from build123d import *

# Parameters (mm, degrees)
BOSS_EXTRUDE1_DEPTH     = 2
BOSS_EXTRUDE2_DEPTH     = 5.4
CUT_EXTRUDE2_DEPTH      = 324.312541101
CUT_EXTRUDE2_DEPTH_BACK = 324.312541101
SKETCH11_R              = 3.15
SKETCH11_R_2            = 8.5
SKETCH13_R              = 3.289472506
BOSS_EXTRUDE3_DEPTH     = 3


with BuildPart() as part:
    # Sketch3 → Boss-Extrude1 (new body)
    with BuildSketch(Plane(origin=(0, 0, 0), x_dir=(1, 0, 0), z_dir=(0, 1, 0))):
        with BuildLine():
            ThreePointArc((271.153533245, 18.921159404), (199.331937646, 37.525228411), (127.510342047, 18.921159404))
            ThreePointArc((127.510342047, 18.921159404), (108.90627304, -52.900436194), (127.510342047, -124.722031793))
            ThreePointArc((127.510342047, -124.722031793), (199.331937646, -143.3261008), (271.153533245, -124.722031793))
            ThreePointArc((271.153533245, -124.722031793), (289.757602252, -52.900436194), (271.153533245, 18.921159404))
        make_face()
    extrude(amount=BOSS_EXTRUDE1_DEPTH)

    # Sketch5 → Boss-Extrude2 (add)
    with BuildSketch(Plane(origin=(0, 2, 0), x_dir=(1, 0, 0), z_dir=(0, 1, 0))):
        with BuildLine():
            Line((121.611565862, -109.080289564), (120.36423024, -109.98653194))
            ThreePointArc((120.36423024, -109.98653194), (108.906273045, -52.899217103), (120.365171108, 4.187908885))
            Line((120.365171108, 4.187908885), (121.612501818, 3.281670078))
            ThreePointArc((121.612501818, 3.281670078), (110.406273045, -52.899216401), (121.611565862, -109.080289564))
        make_face()
        with BuildLine():
            Line((143.152084277, -130.620807978), (142.2458419, -131.8681436))
            ThreePointArc((142.2458419, -131.8681436), (199.331937646, -143.3261008), (256.418033392, -131.8681436))
            Line((256.418033392, -131.8681436), (255.511791015, -130.620807978))
            ThreePointArc((255.511791015, -130.620807978), (199.331937646, -141.8261008), (143.152084277, -130.620807978))
        make_face()
        with BuildLine():
            Line((277.052309429, 3.279417175), (278.299645052, 4.185659552))
            ThreePointArc((278.299645052, 4.185659552), (289.757602252, -52.900436194), (278.299645052, -109.98653194))
            Line((278.299645052, -109.98653194), (277.052309429, -109.080289564))
            ThreePointArc((277.052309429, -109.080289564), (288.257602252, -52.900436194), (277.052309429, 3.279417175))
        make_face()
        with BuildLine():
            Line((255.511791015, 24.819935589), (256.418033392, 26.067271212))
            ThreePointArc((256.418033392, 26.067271212), (199.330718555, 37.525228406), (142.243592567, 26.066330343))
            Line((142.243592567, 26.066330343), (143.149831374, 24.818999633))
            ThreePointArc((143.149831374, 24.818999633), (199.330717853, 36.025228406), (255.511791015, 24.819935589))
        make_face()
    extrude(amount=BOSS_EXTRUDE2_DEPTH)

    # Sketch11 → Cut-Extrude2 (cut, two sides: drawn at the far end of the back side and taken through both)
    with BuildSketch(Plane(origin=(0, 2, 0), x_dir=(1, 0, 0), z_dir=(0, 1, 0)).offset(-CUT_EXTRUDE2_DEPTH_BACK)):
        with Locations(Location((171.047666398, -24.616164947, 0), (0, 0, 270))):
            Circle(SKETCH11_R)
        with Locations(Location((227.616208893, -24.616164947, 0), (0, 0, 270))):
            Circle(SKETCH11_R)
        with Locations(Location((227.616208893, -81.184707442, 0), (0, 0, 270))):
            Circle(SKETCH11_R)
        with Locations(Location((171.047666398, -81.184707442, 0), (0, 0, 270))):
            Circle(SKETCH11_R)
        with Locations(Location((199.331937646, -75.900436194, 0), (0, 0, 270))):
            Circle(SKETCH11_R_2)
    extrude(amount=CUT_EXTRUDE2_DEPTH + CUT_EXTRUDE2_DEPTH_BACK, mode=Mode.SUBTRACT)

    # Sketch13 → Boss-Extrude3 (add)
    with BuildSketch(Plane(origin=(0, 2, 0), x_dir=(1, 0, 0), z_dir=(0, 1, 0))):
        with Locations(Location((189.331937646, -85.900436194, 0), (0, 0, 270))):
            Circle(SKETCH13_R)
        with Locations(Location((209.331937646, -85.900436194, 0), (0, 0, 270))):
            Circle(SKETCH13_R)
    extrude(amount=BOSS_EXTRUDE3_DEPTH)


solid = part.part
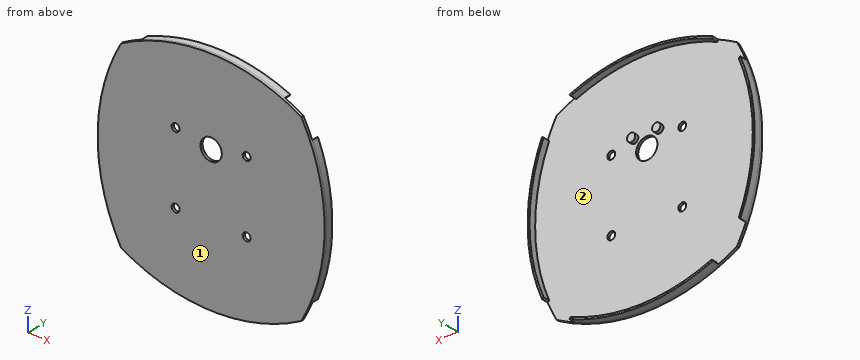
CAD build for the part. Positions are in the model's coordinates, mm. Face numbers are marked on the shaded views. Round coordinates to 2 decimals unless told otherwise and drop trailing zeros. Loops run counter-clockwise (first coordinate to the right, second up) from the corner with the lowest first, then second, coordinate; pieces in that order, holes last.
(1) Wall check: line 1 along Z through (x, y) = (169.5, 1.5); line 2 along X through (y, z) = (6, 50) (3 decimals); line 3 along Z through (x, y) = (187, 3.5). Give the ranges that are in metal, low to high.
(2) Cut at D-D (z = 2). Give the cut face in (x, y).
(3) Drop flat-ended pins along their axis: pin 1 (12 mm diameter, centred on x = 270.5, z = 42.5, fed in from +Y); pin 2 (4 mm diameter, centred on x = 227.62, z = 24.62, fed in from -Y); pin 3 (3.5 mm diameter, centred on x = 208, z = 87, fed in from +Y); pin 4 (2 mm diameter, centred on y = 6, z = 7.5, fed in from -X). Give the stop position or say it passes through.
(4) Cut at B-B (z = 73). Give the cut face in (x, y), plus the area to 3 significant figures.
(5) Cut at A-A (y = 3.5). Give the cut face in (x, z), plus the area to 3 significant figures.
(6) Cut at C-C (x = 250). Give the cut face in (y, z).
(7) Two-plate mould, pull along X, no slides. Class the marked faces 1 and 2: +X half, -X half, draft (parallel to the pull), parting line (faces both ways), or undercut.
Findings below:
1. line 1: z = -34.49 to 21.87, 27.36 to 78.44, 83.93 to 140.29
1. line 2: x = 108.935 to 110.435, 288.229 to 289.729
1. line 3: z = -37.01 to -35.51, 83.58 to 88.22, 141.31 to 142.81
2. outline: (117.94, 0) - (280.73, 0) - (280.73, 7.4) - (279.13, 7.4) - (279.13, 2) - (119.54, 2) - (119.54, 7.4) - (117.94, 7.4) - close
3. pin 1: stops at y = 2
3. pin 2: passes through
3. pin 3: stops at y = 5
3. pin 4: stops at x = 115.73
4. outline: (110.28, 0) - (191.34, 0) - (191.34, 2) - (111.79, 2) - (111.79, 7.4) - (110.28, 7.4) - close; (207.32, 0) - (288.39, 0) - (288.39, 7.4) - (286.87, 7.4) - (286.87, 2) - (207.32, 2) - close
4. area: 341 mm2
5. outline: (120.36, 109.99) arc R147.94 ccw to (120.37, -4.19) - (121.61, -3.28) arc R146.44 cw to (121.61, 109.08) - close; (142.24, -26.07) arc R147.94 ccw to (256.42, -26.07) - (255.51, -24.82) arc R146.44 cw to (143.15, -24.82) - close; (142.25, 131.87) - (143.15, 130.62) arc R146.44 cw to (255.51, 130.62) - (256.42, 131.87) arc R147.94 ccw to start; circle Ø6.58 at (189.33, 85.9); circle Ø6.58 at (209.33, 85.9); (277.05, -3.28) - (278.3, -4.19) arc R147.94 ccw to (278.3, 109.99) - (277.05, 109.08) arc R146.44 cw to start
5. area: 766 mm2
6. outline: (0, -28.58) - (7.4, -28.58) - (7.4, -26.98) - (2, -26.98) - (2, 132.78) - (7.4, 132.78) - (7.4, 134.38) - (0, 134.38) - close
7. face 1: draft
7. face 2: undercut
